Can you work these out from the model? Positions are in its coordinate system, mm. A direction names the side the tool comes from. Round coordinates to 2 decimals unless told otherwise and drop trailing zeros. Loops run counter-clockwise (first coordinate to the right, second up) from the corner with the lowest first, then second, coordinate; pieces in that order, holes last. Notation, with made-up numbers: (59, 4.25) -> (96, 4.25) arc R30 cw to (96, 39.25) -> close; hole circle Ø7 at (15, 25). An arc over 180 degrees is marked (long way). Write item = value, one per line.
from build123d import *

# Parameters (mm, degrees)
SKETCH005_W         = 180
SKETCH005_H         = 85
SKETCH005_R         = 3.75
SKETCH005_W_2       = 110
SKETCH005_H_2       = 30
PAD005_DEPTH        = 10
PAD006_DEPTH        = 6
PAD007_DEPTH        = 6
HOLE005_D           = 5.5
HOLE005_DEPTH       = 25
HOLE005_CBORE_D     = 10
HOLE005_CBORE_DEPTH = 5.4
PAD025_DEPTH        = 30


with BuildPart() as part:
    # Sketch005 → Pad005 (new body)
    with BuildSketch(Plane.XY):
        with Locations((0, 42.5)):
            Rectangle(SKETCH005_W, SKETCH005_H)
        with Locations((-80, 75)):
            Circle(SKETCH005_R, mode=Mode.SUBTRACT)
        with Locations((80, 75)):
            Circle(SKETCH005_R, mode=Mode.SUBTRACT)
        with Locations((-80, 10)):
            Circle(SKETCH005_R, mode=Mode.SUBTRACT)
        with Locations((80, 10)):
            Circle(SKETCH005_R, mode=Mode.SUBTRACT)
        with Locations((0, 35)):
            Rectangle(SKETCH005_W_2, SKETCH005_H_2, mode=Mode.SUBTRACT)
    extrude(amount=PAD005_DEPTH)

    # Sketch006 → Pad006 (join)
    with BuildSketch(Plane.XZ.offset(-20)):
        with BuildLine():
            Line((-55.000007, 9.999997), (-55.000007, 5))
            Line((-55.000007, 5), (54.999984, 5))
            Line((54.999984, 5), (54.999984, 10.000016))
            ThreePointArc((54.999984, 10.000016), (-1.6e-05, 34.078581), (-55.000007, 9.999997))
        make_face()
    extrude(amount=PAD006_DEPTH)

    # Sketch007 → Pad007 (join)
    with BuildSketch(Plane.XZ.offset(-50)):
        with BuildLine():
            Line((-55.000002, 9.999998), (-55.000002, 5))
            Line((-55.000002, 5), (54.999984, 5))
            Line((54.999984, 5), (54.999984, 10.000017))
            ThreePointArc((54.999984, 10.000017), (-1.3e-05, 34.144872), (-55.000002, 9.999998))
        make_face()
    extrude(amount=-PAD007_DEPTH)

    # Hole005
    with Locations(Plane.XY.offset(10)):
        with Locations((-62.5, 12.5), (-62.5, 32.5), (-62.5, 55), (-62.5, 75), (62.5, 12.5), (62.5, 32.5), (62.5, 55), (62.5, 75)):
            CounterBoreHole(HOLE005_D / 2, HOLE005_CBORE_D / 2, HOLE005_CBORE_DEPTH, depth=HOLE005_DEPTH)

    # Sketch046 → Pad025 (join)
    with BuildSketch(Plane.XZ.offset(-20)):
        with BuildLine():
            ThreePointArc((54.919348, 9.999997), (47.923207, 16.740644), (40.107089, 22.510446))
            Line((40.107089, 22.510446), (40.107089, 15.000094))
            Line((40.107089, 15.000094), (54.919348, 0.019657))
            Line((54.919348, 9.999997), (54.919348, 0.019657))
        make_face()
        with BuildLine():
            ThreePointArc((-40.185018, 22.531307), (-48.003192, 16.751155), (-55.000021, 9.999978))
            Line((-55.000021, 0), (-55.000021, 9.999978))
            Line((-40.185018, 15), (-55.000021, 0))
            Line((-40.185018, 22.531307), (-40.185018, 15))
        make_face()
    extrude(amount=-PAD025_DEPTH)


solid = part.part
1. Suppose I cut it at A-A, the plane y = 75. List the corners of the cut face in (x, z) for me.
Entries:
outline = (-90, 0) -> (-83.75, 0) -> (-83.75, 10) -> (-90, 10) -> close; (-76.25, 0) -> (-65.25, 0) -> (-65.25, 4.6) -> (-67.5, 4.6) -> (-67.5, 10) -> (-76.25, 10) -> close; (-59.75, 0) -> (59.75, 0) -> (59.75, 4.6) -> (57.5, 4.6) -> (57.5, 10) -> (-57.5, 10) -> (-57.5, 4.6) -> (-59.75, 4.6) -> close; (65.25, 0) -> (76.25, 0) -> (76.25, 10) -> (67.5, 10) -> (67.5, 4.6) -> (65.25, 4.6) -> close; (83.75, 0) -> (90, 0) -> (90, 10) -> (83.75, 10) -> close
2. I'm going to push flat-ended pins straight in: pin 1 (2 mm diameter, centred on y = 29.5, z = 15, fed in from +X); pin 2 (11 mm diameter, centred on x = -61, y = 73.5, fed in from +Z); pin 3 (8 mm diameter, centred on x = 62.5, y = 12.5, fed in from +Z). Where does each tip first touch, or does it pass through?
Entries:
pin_1 = 50.99
pin_2 = 10
pin_3 = 4.6
3. For faces 1 (the flat face through (-60, 53, 4.6)), 2 (the flat face through (-1, 14, 20)), 3 (the flat face through (-40.185, 35, 19)), 4 (the flat face through (-47.489, 34.79, 7.605)), which set-ups out of +Z, -Z, +X, -X, +Y, -Y let a thin tool reach every point of the face, with its end or its side?
Entries:
face_1 = +Z
face_2 = +Z, +X, -X, -Y
face_3 = +Z, -Z
face_4 = -Z
4. I need wall thicknesses on line 1 (Y direction, x = -62.5, z = 3.45); line 2 (Y direction, x = 62.5, z = 8.35); line 3 (Y direction, x = 80, z = 6). Which ranges of each line are inside material? Lowest first, please. Write a range as [from, to].
Entries:
line_1 = [0, 9.75], [15.25, 29.75], [35.25, 52.25], [57.75, 72.25], [77.75, 85]
line_2 = [0, 7.5], [17.5, 27.5], [37.5, 50], [60, 70], [80, 85]
line_3 = [0, 6.25], [13.75, 71.25], [78.75, 85]
5. Suppose I cut it at D-D, the plane x = -11.5. List the corners of the cut face in (y, z) for me.
Entries:
outline = (0, 0) -> (20, 0) -> (20, 33.19) -> (14, 33.19) -> (14, 10) -> (0, 10) -> close; (50, 0) -> (85, 0) -> (85, 10) -> (56, 10) -> (56, 33.25) -> (50, 33.25) -> close
6. Suppose I cut it at B-B, the plane x = 80. List the corners of the cut face in (y, z) for me.
Entries:
outline = (0, 0) -> (6.25, 0) -> (6.25, 10) -> (0, 10) -> close; (13.75, 0) -> (71.25, 0) -> (71.25, 10) -> (13.75, 10) -> close; (78.75, 0) -> (85, 0) -> (85, 10) -> (78.75, 10) -> close
7. Suppose I cut it at C-C, the plane y = 48. Count the separate pieces of the cut face and the enclosed holes in it, and give its area (3 significant figures).
Entries:
separate_pieces = 3
enclosed_holes = 0
area = 976 mm²
